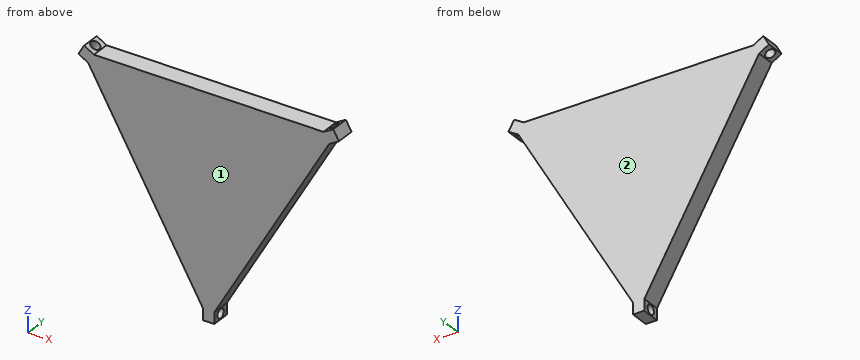
from build123d import *

# Parameters (mm, degrees)
BOSS_EXTRUDE1_DEPTH = 10
SKETCH2_R           = 2.5
CUT_EXTRUDE1_DEPTH  = 134.326025
SKETCH3_R           = 2.5
CUT_EXTRUDE2_DEPTH  = 6


with BuildPart() as part:
    # Sketch1 → Boss-Extrude1 (new body)
    with BuildSketch(Plane(origin=(0, 0, 0), x_dir=(1, 0, 0), z_dir=(0, 1, 0))):
        Polygon((-3, 110.383597966), (-63.73, 5.196152423), (-68.926152423, 2.196152423), (-65.926152423, -3), (-60.73, 0), (60.73, 0), (65.926152423, -3), (68.926152423, 2.196152423), (63.73, 5.196152423), (3, 110.383597966), (3, 116.383597966), (-3, 116.383597966), align=None)
    extrude(amount=BOSS_EXTRUDE1_DEPTH)

    # Sketch2 → Cut-Extrude1 (cut)
    with BuildSketch(Plane(origin=(-15.1825, 0, -26.296861386), x_dir=(0.866025404, 0, -0.5), z_dir=(0.5, 0, 0.866025404))):
        with Locations((-55.593722772, 5)):
            Circle(SKETCH2_R)
    cut_extrude1 = extrude(amount=-CUT_EXTRUDE1_DEPTH, mode=Mode.SUBTRACT)

    # Mirror6: Cut-Extrude1 across plane
    add(cut_extrude1.mirror(Plane.ZY), mode=Mode.SUBTRACT)

    # Sketch3 → Cut-Extrude2 (cut)
    with BuildSketch(Plane.ZY.offset(2.999999999)):
        with Locations((-113.383597966, 5)):
            Circle(SKETCH3_R)
    extrude(amount=-CUT_EXTRUDE2_DEPTH, mode=Mode.SUBTRACT)


solid = part.part
Can you work these out from the model? Positions are in its coordinate system, mm. Face numbers are marked on the shaded views. Round coordinates to 2 decimals unless told otherwise and drop trailing zeros. Write each loop counter-clockwise with the first axis right and the second up, starting at its lowest first coordinate (ties: lowest second). Pieces come first, ordered by that corner, then holes. Notation, with made-up numbers: (80.25, 16.5) -> (101.25, 16.5) arc R22 cw to (101.25, 37.5) -> close; hole circle Ø9 at (55, 40). An arc over 180 degrees is marked (long way). One line per question, with ' | ' between items. Start each with the question number.
1) I need wall thicknesses on line 1 (Z direction, x = 2, y = 6.25); line 2 (X direction, y = 0.5, z = -92.5); line 3 (X direction, y = 3.25, z = -22). Which ranges of each line are inside material? Lowest first, please. Write a range as [from, to].
2) If we mould it in two halves opening along Y, with no side actions, what happens to the marked faces 1 and 2? For each: released by +Y, released by -Y, zero draft, split by the parting line, or undercut.
3) Suppose I cut it at A-A on y = 5. Write out the boundary of the cut face in (x, z), then the cut area to 3 significant figures.
4) I'm going to push flat-ended pins straight in: P1, Ø1.8, axis at y = 7, z = -112, coming from the +X side; P2, Ø1.5, axis at x = 21, y = 2, coming from the -Z side; P3, Ø5, axis at y = 3.5, z = -114, coming from the -X side. Where does each tip first touch, or does it pass through?
5) Suppose I cut it at B-B on x = -47. Write out the boundary of the cut face in (y, z).
6) Suppose I cut it at C-C on z = -16. Write out the boundary of the cut face in (x, y), then the cut area to 3 significant figures.
Return value:
1) line 1: z = [-116.38, -115.55], [-111.22, 0] | line 2: x = [-13.33, 13.33] | line 3: x = [-54.03, 54.03]
2) face 1: released by -Y | face 2: released by +Y
3) outline: (-68.93, -2.2) -> (-68.49, -2.45) -> (-65.49, 2.75) -> (-65.93, 3) -> close; (-64.16, -4.95) -> (-63.73, -5.2) -> (-3, -110.38) -> (-3, -110.88) -> (3, -110.88) -> (3, -110.38) -> (63.73, -5.2) -> (64.16, -4.95) -> (61.16, 0.25) -> (60.73, 0) -> (-60.73, 0) -> (-61.16, 0.25) -> close; (-3, -116.38) -> (3, -116.38) -> (3, -115.88) -> (-3, -115.88) -> close; (65.49, 2.75) -> (68.49, -2.45) -> (68.93, -2.2) -> (65.93, 3) -> close | area: 7,680 mm2
4) P1: stops at x = 3 | P2: stops at z = -80.51 | P3: stops at x = -3
5) outline: (0, -34.17) -> (10, -34.17) -> (10, 0) -> (0, 0) -> close
6) outline: (-57.49, 0) -> (57.49, 0) -> (57.49, 10) -> (-57.49, 10) -> close | area: 1,150 mm2
